Design review of the part built by this model. Coordinates are the model's own, in mm. A direction names the side the tool comes from. Give positions to 0.01 mm unless a question says otherwise; leave off trailing zeros. Loops run counter-clockwise (first coordinate to the right, second up) from the corner with the lowest first, then second, coordinate; pieces in that order, holes last.
Autodesk Inventor part; units mm, degrees
ref_plane "YZ Plane" through (0, 0, 0) normal (1, 0, 0) x (0, 1, 0)
ref_plane "XZ Plane" through (0, 0, 0) normal (0, 1, 0) x (-1, 0, 0)
ref_plane "XY Plane" through (0, 0, 0) normal (0, 0, 1) x (1, 0, 0)
ref_plane "Work Plane1" through (0, 0, 0) normal (0, 0, 1) x (1, 0, 0)
sketch "Sketch1" plane through (0, 0, 0) normal (0, 0, 1) x (1, 0, 0)
  circle A0 centre (0, -55.5) radius 5.1943
  circle A1 centre (-55.5, 0) radius 5.1943
  circle A2 centre (0, 55.5) radius 5.1943
  circle A3 centre (55.5, 0) radius 5.1943
  circle A4 centre (0, 0) radius 61.5
  circle A5 centre (0, 0) radius 49.5
  line L0 (-2.0207, 52) -> (-4.0415, 55.5)
  line L1 (-4.0415, 55.5) -> (-2.0207, 59)
  line L2 (-2.0207, 59) -> (2.0207, 59)
  line L3 (2.0207, 59) -> (4.0415, 55.5)
  line L4 (4.0415, 55.5) -> (2.0207, 52)
  line L5 (2.0207, 52) -> (-2.0207, 52)
  line L6 (0, 55.5) -> (0, 52) construction
  line L7 (-52, -2.0207) -> (-55.5, -4.0415)
  line L8 (-55.5, -4.0415) -> (-59, -2.0207)
  line L9 (-59, -2.0207) -> (-59, 2.0207)
  line L10 (-59, 2.0207) -> (-55.5, 4.0415)
  line L11 (-55.5, 4.0415) -> (-52, 2.0207)
  line L12 (-52, 2.0207) -> (-52, -2.0207)
  line L13 (2.0207, -52) -> (4.0415, -55.5)
  line L14 (4.0415, -55.5) -> (2.0207, -59)
  line L15 (2.0207, -59) -> (-2.0207, -59)
  line L16 (-2.0207, -59) -> (-4.0415, -55.5)
  line L17 (-4.0415, -55.5) -> (-2.0207, -52)
  line L18 (-2.0207, -52) -> (2.0207, -52)
  line L19 (52, 2.0207) -> (55.5, 4.0415)
  line L20 (55.5, 4.0415) -> (59, 2.0207)
  line L21 (59, 2.0207) -> (59, -2.0207)
  line L22 (59, -2.0207) -> (55.5, -4.0415)
  line L23 (55.5, -4.0415) -> (52, -2.0207)
  line L24 (52, -2.0207) -> (52, 2.0207)
  circle A6 centre (0, 55.5) radius 5.1943
  circle A7 centre (-39.2444, 39.2444) radius 5.1943
  line L25 (-39.2444, 39.2444) -> (0, 0)
  line L26 (0, 55.5) -> (0, -55.5)
  circle A8 centre (-39.2444, -39.2444) radius 5.1943
  circle A9 centre (39.2444, -39.2444) radius 5.1943
  circle A10 centre (39.2444, 39.2444) radius 5.1943
  circle A11 centre (0, -55.5) radius 2
  circle A12 centre (55.5, 0) radius 2
  circle A13 centre (0, 55.5) radius 2
  circle A14 centre (-55.5, 0) radius 2
  point P0 (-52, 0)
  point P1 (0, -52)
  point P2 (52, 0)
  dimension "d2" = 7
  dimension "d5" = 360
  dimension "d11" = 45
  dimension "d12" = 10.3886
  dimension "d13" = 55.5
  dimension "d16" = 360
  dimension "d32" = 4
  dimension "d35" = 360
extrude "Extrusion1" add sketch "Sketch1" along normal blind 8.89 contours A11 | L18 L13 L14 L15 L16 L17 | A0 | A7 | A13 | L5 L0 L1 L2 L3 L4 | A2 | A1 | A3 | A4 | L7 L8 L9 L10 L11 L12 | L19 L20 L21 L22 L23 L24 | A8 | A9 | A10 | A12 | A14
extrude "Extrusion2" cut sketch "Sketch1" along normal blind 6.35 contours A11 | L18 L13 L14 L15 L16 L17 | A13 | L5 L0 L1 L2 L3 L4 | L7 L8 L9 L10 L11 L12 | L19 L20 L21 L22 L23 L24 | A12 | A14
sketch "Sketch2" plane through (0, 0, 8.89) normal (0, 0, 1) x (1, 0, 0)
  circle A0 centre (39.2444, 39.2444) radius 5.1943
  circle A1 centre (39.2444, -39.2444) radius 5.1943
  circle A2 centre (-39.2444, -39.2444) radius 5.1943
  circle A3 centre (-39.2444, 39.2444) radius 5.1943
  circle A4 centre (39.2444, -39.2444) radius 4
  circle A5 centre (0, 0) radius 49.5
  circle A6 centre (39.2444, 39.2444) radius 4
  circle A7 centre (-39.2444, 39.2444) radius 4
  circle A8 centre (-39.2444, -39.2444) radius 4
  circle A9 centre (39.2444, -39.2444) radius 2
  circle A10 centre (39.2444, 39.2444) radius 2
  circle A11 centre (-39.2444, 39.2444) radius 2
  circle A12 centre (-39.2444, -39.2444) radius 2
  dimension "d18" = 8
  dimension "d21" = 360
  dimension "d25" = 4
  dimension "d28" = 360
extrude "Extrusion3" cut sketch "Sketch2" against normal blind 6.35 contours A4 | A6 | A7 | A8 | A9 | A10 | A11 | A12
extrude "Extrusion4" cut sketch "Sketch2" against normal blind 15.875 contours A9 | A10 | A11 | A12
extrude "Extrusion5" cut sketch "Sketch1" along normal through all contours A11 | A13 | A12 | A14
properties part number "TopSpacer"
Q1. Insertion check: pin 1 (3 mm diameter, centred on x = 10, z = 2.5, fed in from +Y); pin 2 (2.5 mm diameter, centred on x = 0, y = 55.5, fed in from +Z); pin 3 (1.2 mm diameter, centred on x = -0.5, z = 4.5, fed in from -Y); pin 4 (4 mm diameter, centred on x = 6, z = 5, fed in from -Y). Each pin has a flat end and moves straight along its axis. Give the tip position at first contact, or say it passes through.
Results:
pin 1: stops at y = 60.91
pin 2: passes through
pin 3: stops at y = -61.5
pin 4: stops at y = -61.37
Q2. Wall thickness on line 1 (Y direction, x = 38.5, z = 8.25); line 2 (X direction, y = -37, z = 5.5); line 3 (X direction, y = 26.5, z = 2): over which ranges is each line inside the solid? List them lowest first.
Results:
line 1: y = -47.96 to -43.17, -35.31 to -31.11, 31.11 to 35.31, 43.17 to 47.96
line 2: x = -49.12 to -42.56, -35.93 to -32.88, 32.88 to 35.93, 42.56 to 49.12
line 3: x = -55.5 to -41.81, 41.81 to 55.5
Q3. Take a section at C-C (y = 16.5). Give the boundary of the cut face in (x, z).
Results:
outline: (-59.25, 0) - (-46.67, 0) - (-46.67, 8.89) - (-59.25, 8.89) - close; (46.67, 0) - (59.25, 0) - (59.25, 8.89) - (46.67, 8.89) - close
Q4. Take a section at B-B (y = -20). Give the boundary of the cut face in (x, z), plus the area to 3 significant figures.
Results:
outline: (-58.16, 0) - (-45.28, 0) - (-45.28, 8.89) - (-58.16, 8.89) - close; (45.28, 0) - (58.16, 0) - (58.16, 8.89) - (45.28, 8.89) - close
area: 229 mm2
Q5. Take a section at A-A (x = 0). Give the boundary of the cut face in (y, z).
Results:
outline: (-61.5, 0) - (-59, 0) - (-59, 6.35) - (-57.5, 6.35) - (-57.5, 8.89) - (-61.5, 8.89) - close; (-53.5, 6.35) - (-52, 6.35) - (-52, 0) - (-49.5, 0) - (-49.5, 8.89) - (-53.5, 8.89) - close; (49.5, 0) - (52, 0) - (52, 6.35) - (53.5, 6.35) - (53.5, 8.89) - (49.5, 8.89) - close; (57.5, 6.35) - (59, 6.35) - (59, 0) - (61.5, 0) - (61.5, 8.89) - (57.5, 8.89) - close
Q6. Tool access review of faces 1 (the face through (-3, -57.3, 3.1)), 2 (the face through (43.06, 40.45, 5.76)), 3 (the face through (-0.26, -57.483, 7.602)): name each direction out of +Z, -Z, +X, -X, +Y, -Y from which nothing blocks a thin tool from reaching the whole face with its end or side.
Results:
face 1: -Z
face 2: +Z
face 3: +Z, -Z
